Geometry: final body of the model. Coordinates: model frame, mm. Give positions to 0.01 mm unless a question says otherwise; leave off trailing zeros. Order: outer loops, then holes, each group sorted by start corner. A loop starts at its lowest first (then second) coordinate and runs counter-clockwise, first axis right, second up. Notation, with made-up numbers: (-19, 27) -> (12, 27) arc R16 cw to (12, 51) -> close; hole circle Ø9 at (68, 32.25). An arc over 180 degrees is marked (long way). One line per question, with ' | ' between items.
from build123d import *

# Parameters (mm, degrees)
F0_R     = 15.875
F1_DEPTH = 3
F3_DEPTH = 5
F4_R     = 2.1
F5_DEPTH = 3


with BuildPart() as f1:
    # F0 (on Top) → F1 (new body)
    with BuildSketch(Plane.XY):
        Circle(F0_R)
    extrude(amount=F1_DEPTH)

    # F2 (on face) → F3 (cut)
    with BuildSketch(Plane.XY.offset(3)):
        with BuildLine():
            ThreePointArc((-5.83022, 8.124563), (-6.798257, 7.333737), (-7.66007, 6.428322))
            ThreePointArc((-7.66007, 6.428322), (-6.305696, 6.184876), (-5.548257, 7.333737))
            ThreePointArc((-5.548257, 7.333737), (-5.620856, 7.753532), (-5.83022, 8.124563))
        make_face()
        with BuildLine():
            ThreePointArc((-5.83022, 8.124563), (-7.648039, 8.250455), (-7.66007, 6.428322))
            ThreePointArc((-7.66007, 6.428322), (-6.798257, 7.333737), (-5.83022, 8.124563))
        make_face()
        with BuildLine():
            ThreePointArc((8.583737, 6.798257), (7.797812, 7.958918), (6.428322, 7.66007))
            ThreePointArc((6.428322, 7.66007), (7.333737, 6.798257), (8.124563, 5.83022))
            ThreePointArc((8.124563, 5.83022), (8.463125, 6.262548), (8.583737, 6.798257))
        make_face()
        with BuildLine():
            ThreePointArc((8.124563, 5.83022), (7.333737, 6.798257), (6.428322, 7.66007))
            ThreePointArc((6.428322, 7.66007), (6.41702, 5.948475), (8.124563, 5.83022))
        make_face()
        with BuildLine():
            ThreePointArc((7.66007, -6.428322), (6.798257, -7.333737), (5.83022, -8.124563))
            ThreePointArc((5.83022, -8.124563), (7.218051, -8.511138), (8.048257, -7.333737))
            ThreePointArc((8.048257, -7.333737), (7.947119, -6.841176), (7.66007, -6.428322))
        make_face()
        with BuildLine():
            ThreePointArc((7.66007, -6.428322), (5.948475, -6.41702), (5.83022, -8.124563))
            ThreePointArc((5.83022, -8.124563), (6.798257, -7.333737), (7.66007, -6.428322))
        make_face()
        with BuildLine():
            ThreePointArc((-6.428322, -7.66007), (-7.333737, -6.798257), (-8.124563, -5.83022))
            ThreePointArc((-8.124563, -5.83022), (-8.250455, -7.648039), (-6.428322, -7.66007))
        make_face()
        with BuildLine():
            ThreePointArc((-6.428322, -7.66007), (-6.173076, -7.262331), (-6.083737, -6.798257))
            ThreePointArc((-6.083737, -6.798257), (-6.798029, -5.668869), (-8.124563, -5.83022))
            ThreePointArc((-8.124563, -5.83022), (-7.333737, -6.798257), (-6.428322, -7.66007))
        make_face()
    extrude(amount=-F3_DEPTH, mode=Mode.SUBTRACT)

    # F4 (on face) → F5 (cut, through all)
    with BuildSketch(Plane.XY.offset(3)):
        Circle(F4_R)
    extrude(amount=-F5_DEPTH, mode=Mode.SUBTRACT)


solid = f1.part
1) Material intervals for probe 1 along Y at (x, z) = (0, 2.45) (3 decimals); probe 2 along X at (y, z) = (-6, 0.25); probe 3 along X at (y, z) = (7.5, 0.4), sorted ascending. Write a range as from..to.
Check result:
probe 1: y = -15.875..-2.1, 2.1..15.875 | probe 2: x = -14.7..-8.3, -6.37..14.7 | probe 3: x = -13.99..-8.04, -5.56..6.3, 8.37..13.99
2) Section C-C on z = 2.35. Return loops of the section in (x, y) (3 decimals), plus the area to 3 significant figures.
Check result:
outline: circle Ø31.75 at (0, 0); hole (-6.428, -7.66) arc R1.25 ccw to (-6.084, -6.798) arc R1.25 ccw (long way) to start; hole (-5.83, 8.125) arc R1.25 ccw (long way) to (-5.548, 7.334) arc R1.25 ccw to start; hole circle Ø4.2 at (0, 0); hole (7.66, -6.428) arc R1.25 ccw (long way) to (8.048, -7.334) arc R1.25 ccw to start; hole (8.125, 5.83) arc R1.25 ccw to (8.584, 6.798) arc R1.25 ccw (long way) to start | area: 758 mm^2
3) Section A-A on y = 0. Return loops of the section in (x, z) (3 decimals).
Check result:
outline: (-15.875, 0) -> (-2.1, 0) -> (-2.1, 3) -> (-15.875, 3) -> close; (2.1, 0) -> (15.875, 0) -> (15.875, 3) -> (2.1, 3) -> close
4) Contact query for a flat-ended pin moving along its axis: pin 1 Ø4 at (x, y) = (7.5, -1) entering from -Z. Output: stop coordinate, or through.
Check result:
pin 1: stops at z = 0
5) Pull-direction query (X, two-part tool) for faces 1 (the cylindrical face through (-3.441, -15.497, 1.479)), 2 (the cylindrical face through (2.003, 0.631, 1.521)), 3 (the flat face through (3, 0, 3)); classes: +X half, -X half, draft (parallel to the pull), parting line (faces both ways), or undercut.
Check result:
face 1: parting line | face 2: undercut | face 3: draft
6) Section D-D on y = 13. Return loops of the section in (x, z).
Check result:
outline: (-9.11, 0) -> (9.11, 0) -> (9.11, 3) -> (-9.11, 3) -> close
